Design review of the part built by this model. Coordinates are the model's own, in mm. A direction names the side the tool comes from. Coordinates: 2 decimals unless noted, no trailing zeros. Write each loop counter-clockwise with the first axis right and the second up, starting at its lowest first coordinate (ties: lowest second). Pieces come first, ordered by that corner, then holes. Notation, with made-up numbers: (-24.75, 53.25) - (-20.75, 53.25) arc R25 cw to (-20.75, 88.25) - close; hole circle Ø11 at (-9.75, 5). An arc over 180 degrees is marked (long way). Answer as a JSON object with one key per item and string values.
```python
from build123d import *

# Parameters (mm, degrees)
BOSS_EXTRUDE1_DEPTH = 2
SKETCH2_W           = 3
SKETCH2_H           = 7.5
BOSS_EXTRUDE2_DEPTH = 15
CUT_EXTRUDE1_REACH  = 4
SKETCH3_R           = 1.625
SKETCH4_R           = 2.35
CUT_EXTRUDE2_DEPTH  = 26.1
FILLET1_R           = 4
FILLET2_R           = 0.5


with BuildPart() as part:
    # Sketch1 → Boss-Extrude1 (new body)
    with BuildSketch(Plane(origin=(0, 0, 0), x_dir=(1, 0, 0), z_dir=(0, 1, 0))):
        Polygon((0, 0), (0, 45), (42, 45), (42, 8), (22, 8), (22, 0), align=None)
    extrude(amount=BOSS_EXTRUDE1_DEPTH)

    # Sketch2 → Boss-Extrude2 (add)
    with BuildSketch(Plane(origin=(0, 2, 0), x_dir=(1, 0, 0), z_dir=(0, 1, 0))):
        with Locations((18.4, 41.25)):
            Rectangle(SKETCH2_W, SKETCH2_H)
        with Locations((18.4, 3.75)):
            Rectangle(SKETCH2_W, SKETCH2_H)
        Polygon((22.1, 45), (22.1, 40), (24.1, 40), (24.1, 37.5), (28.1, 37.5), (28.1, 45), align=None)
    extrude(amount=BOSS_EXTRUDE2_DEPTH)

    # Sketch3 → Cut-Extrude1 (cut, up to next)
    with BuildSketch(Plane(origin=(0, 2, 0), x_dir=(1, 0, 0), z_dir=(0, 1, 0)), mode=Mode.PRIVATE) as cut_extrude1_sk1:
        with Locations((11.45, 40.5)):
            Circle(SKETCH3_R)
    cut_extrude1_tool1 = extrude(cut_extrude1_sk1.sketch, amount=-CUT_EXTRUDE1_REACH, mode=Mode.PRIVATE) & part.part
    add(cut_extrude1_tool1.solids().sort_by_distance((11.45, 2, -40.5))[0], mode=Mode.SUBTRACT)
    # Sketch3 → Cut-Extrude1 (cut, up to next)
    with BuildSketch(Plane(origin=(0, 2, 0), x_dir=(1, 0, 0), z_dir=(0, 1, 0)), mode=Mode.PRIVATE) as cut_extrude1_sk2:
        with Locations((11.45, 4.5)):
            Circle(SKETCH3_R)
    cut_extrude1_tool2 = extrude(cut_extrude1_sk2.sketch, amount=-CUT_EXTRUDE1_REACH, mode=Mode.PRIVATE) & part.part
    add(cut_extrude1_tool2.solids().sort_by_distance((11.45, 2, -4.5))[0], mode=Mode.SUBTRACT)

    # Sketch4 → Cut-Extrude2 (cut, through all)
    with BuildSketch(Plane(origin=(16.9, 0, 0), x_dir=(0, 0, -1), z_dir=(1, 0, 0))):
        with Locations((40.155, 8.58)):
            Circle(SKETCH4_R)
        with Locations((4.845, 8.58)):
            Circle(SKETCH4_R)
    extrude(amount=CUT_EXTRUDE2_DEPTH, mode=Mode.SUBTRACT)

    # Fillet1
    fillet1_edges = [part.edges().sort_by_distance(p)[0] for p in [
        (16.9, 2, -3.75),
        (16.9, 2, -41.25),
        (28.1, 2, -41.25),
    ]]
    fillet(fillet1_edges, radius=FILLET1_R)

    # Fillet2
    fillet2_edges = [part.edges().sort_by_distance(p)[0] for p in [
        (19.9, 2, -3.75),
        (19.9, 2, -41.25),
        (22.1, 2, -42.5),
    ]]
    fillet(fillet2_edges, radius=FILLET2_R)


solid = part.part
```
(1) Take a section at A-A, the plane y = 8.58. Write out the cut boundary in (x, z) (3 decimals), and give its area (3 significant figures).
Solved:
{"outline": "(16.9, -45) - (19.9, -45) - (19.9, -42.505) - (16.9, -42.505) - close; (16.9, -37.805) - (19.9, -37.805) - (19.9, -37.5) - (16.9, -37.5) - close; (16.9, -7.5) - (19.9, -7.5) - (19.9, -7.195) - (16.9, -7.195) - close; (16.9, -2.495) - (19.9, -2.495) - (19.9, 0) - (16.9, 0) - close; (22.1, -45) - (28.1, -45) - (28.1, -42.505) - (22.1, -42.505) - close; (24.1, -37.805) - (28.1, -37.805) - (28.1, -37.5) - (24.1, -37.5) - close", "area": "33.0 mm^2"}
(2) Take a section at D-D, the plane x = 21. Write out the cut boundary in (y, z).
Solved:
{"outline": "(0, -45) - (2, -45) - (2, 0) - (0, 0) - close"}
(3) Take a section at C-C, the plane y = 15.5. Write out the cut boundary in (x, z), and give its area (3 significant figures).
Solved:
{"outline": "(16.9, -45) - (19.9, -45) - (19.9, -37.5) - (16.9, -37.5) - close; (16.9, -7.5) - (19.9, -7.5) - (19.9, 0) - (16.9, 0) - close; (22.1, -45) - (28.1, -45) - (28.1, -37.5) - (24.1, -37.5) - (24.1, -40) - (22.1, -40) - close", "area": "85.0 mm^2"}
(4) For pin 1 (12.5 mm diameter, centred on x = 14.5, z = -24, fed in from +Y); pin 2 (9 mm diameter, centred on x = 26, y = 12.5, fed in from +Z); pin 3 (1.5 mm diameter, centred on y = 7.5, z = -42.5, fed in from -X), all flat-tipped, find the tip position at first contact; note any pin that passes through.
Solved:
{"pin 1": "stops at y = 2", "pin 2": "stops at z = -37.5", "pin 3": "stops at x = 16.9"}
(5) To check wall thickness, follow line 1 (Z direction, x = 11.45, y = 0.5) (3 decimals); line 2 (Z direction, x = 17.5, y = 8.58) (3 decimals); line 3 (Y direction, x = 33, z = -41). State the ranges of each line that lie inside material, in increasing order. Write a range as from..to.
Solved:
{"line 1": "z = -45..-42.125, -38.875..-6.125, -2.875..0", "line 2": "z = -45..-42.505, -37.805..-37.5, -7.5..-7.195, -2.495..0", "line 3": "y = 0..2"}
(6) The part is to be moulded in two halves that separate along X. For faces 4 (the face through (19.9, 11, -41)), 5 (the face through (42, 1, -27)), 6 (the face through (0, 1, -22)), 7 (the face through (18, 9, -7.5)), say which applies: pulls with the +X half, pulls with the -X half, needs draft (parallel to the pull), parting line crosses it, or undercut.
Solved:
{"face 4": "undercut", "face 5": "pulls with the +X half", "face 6": "pulls with the -X half", "face 7": "needs draft"}
(7) Take a section at B-B, the plane x = 11.45. Write out the cut boundary in (y, z) (3 decimals).
Solved:
{"outline": "(0, -45) - (2, -45) - (2, -42.125) - (0, -42.125) - close; (0, -38.875) - (2, -38.875) - (2, -6.125) - (0, -6.125) - close; (0, -2.875) - (2, -2.875) - (2, 0) - (0, 0) - close"}
(8) Tool access review of faces 1 (the face through (19.9, 11, -4)), 2 (the face through (26, 9, -37.5)), 3 (the face through (16.9, 13, -4)): name each direction out of +Z, -Z, +X, -X, +Y, -Y from which nothing blocks a thin tool from reaching the whole face with its end or side.
Solved:
{"face 1": "+Z, -Z, +X, +Y", "face 2": "+Z, +X, -X, +Y", "face 3": "+Z, -Z, -X, +Y"}
